Here's how the part is built. I have some questions about the finished solid (model axes, mm). A direction names the side the tool comes from. Round coordinates to 2 decimals unless told otherwise and drop trailing zeros. Loops run counter-clockwise (first coordinate to the right, second up) from the corner with the lowest first, then second, coordinate; pieces in that order, holes last. Notation, with made-up numbers: (42, -5) - (98, -5) arc R19 cw to (98, 28) - close; hole circle Ø2 at (44, 79.25). An arc over 180 degrees is marked (long way). Answer as a JSON object with one key per item and string values. Group by question number.
1) If I drill on line 1 along Z through (x, y) = (-50, -0.25); line 2 along X through (y, z) = (7, 1); line 3 along X through (y, z) = (5, -2.5), over which ranges is the centre line in solid material (lowest first)? Write a range as [from, to].
2) Will these pins go through, and if not, where does the flat tip stop? P1, Ø4, axis at y = 6, z = -2, coming from the -X side; P2, Ø6, axis at x = -46.5, z = 2.5, coming from the +Y side; P3, Ø8, axis at x = -12.5, y = -6.5, coming from the +Z side; P4, Ø1, axis at x = -39.5, y = 6, coming from the +Z side.
3) I want a section at B-B, the plane x = -13.5. Please give me the cut outline in (y, z) (1 decimal), then the cut area to 3 significant figures.
4) Which directions (+Z, -Z, +X, -X, +Y, -Y) give clear straight access to the entire face, cutting with the end or side of a thin tool? Please do faces 1 (the face through (3.04, 6.17, 3.49)), 2 (the face through (-34.25, 4.65, 1.03)).
5) I want a section at A-A, the plane y = 0. Please give me the cut outline in (x, z).
from build123d import *

# Parameters (mm, degrees)
HEX_HEAD_DEPTH  = 6.35
SKETCH3_R       = 4.7625
BOLT_BODY_DEPTH = 69.85
CHAMFER1_SIZE   = 0.762
FILLET1_R       = 0.381


with BuildPart() as part:
    # Sketch1 → HEX-HEAD (new body)
    with BuildSketch(Plane(origin=(0, 0, 0), x_dir=(0, 0, -1), z_dir=(1, 0, 0))):
        Polygon((0, 8.182900835), (-7.0866, 4.091450418), (-7.0866, -4.091450418), (0, -8.182900835), (7.0866, -4.091450418), (7.0866, 4.091450418), align=None)
    extrude(amount=HEX_HEAD_DEPTH)

    # Sketch2 → EDGE-CUT (revolve, cut)
    with BuildSketch(Plane.XY, mode=Mode.PRIVATE) as edge_cut_sk:
        Polygon((6.35, 6.658900835), (5.67731061, 8.182900835), (6.35, 8.182900835), align=None)
    revolve(edge_cut_sk.sketch.rotate(Axis((0, 0, 0), (1, 0, 0)), 90), axis=Axis((0, 0, 0), (1, 0, 0)), mode=Mode.SUBTRACT)

    # Sketch3 → BOLT-BODY (add)
    with BuildSketch(Plane.ZY):
        with Locations(Location((0, 0, 0), (0, 0, 180))):
            Circle(SKETCH3_R)
    extrude(amount=BOLT_BODY_DEPTH)

    # Chamfer1
    chamfer1_edges = [part.edges().sort_by_distance(p)[0] for p in [
        (-69.85, 0, 4.7625),
    ]]
    chamfer(chamfer1_edges, length=CHAMFER1_SIZE)

    # Fillet1
    fillet1_edges = [part.edges().sort_by_distance(p)[0] for p in [
        (0, 0, 4.7625),
    ]]
    fillet(fillet1_edges, radius=FILLET1_R)


solid = part.part
Outcome:
{
 "1": {"line 1": "[-4.76, 4.76]", "line 2": "[0, 6.17]", "line 3": "[0, 6.35]"},
 "2": {"P1": "x = -69.53", "P2": "y = 4.76", "P3": "z = 4.05", "P4": "through"},
 "3": {"outline": "circle Ø9.5 at (0, 0)", "area": "71.3 mm^2"},
 "4": {"face 1": "+Z, +X, -X, +Y", "face 2": "-X"},
 "5": {"outline": "(-69.85, -4) - (-69.09, -4.76) - (-0.38, -4.76) arc R0.38 cw to (0, -5.14) - (0, -7.09) - (6.16, -7.09) - (6.35, -6.66) - (6.35, 6.66) - (6.16, 7.09) - (0, 7.09) - (0, 5.14) arc R0.38 cw to (-0.38, 4.76) - (-69.09, 4.76) - (-69.85, 4) - close"}
}
